The listing builds one solid part. Answer for the finished solid, in the listing's coordinates (mm). A direction names the side the tool comes from. Give positions to 0.01 mm unless a question says otherwise; leave off trailing zeros. Order: outer loops, then holes, each group sorted by start corner. A loop starts at its lowest first (then second) coordinate and runs counter-clockwise, first axis right, second up. Notation, with made-up numbers: (-9.5, -7.75) - (43.5, -7.75) arc R15 ccw to (43.5, 8.25) - close; hole circle Ø7 at (-4.5, 32.5). An arc over 180 degrees is marked (long way). Write each question's results on one line, items separated by ' | '. Start each with the question number.
1. Section C-C (x = -3) is taken. Give the vertices of the cut face in (y, z).
2. Find the intervals of material crossed by L1, parallel to X at y = 3.25, z = 9.5; L2, parallel to Z at x = 15, y = 13.5; L3, parallel to Y at x = 59, z = 8, in increasing order.
3. Which of the six approach directions +Z, -Z, +X, -X, +Y, -Y give full straight-line access (tool end or side, diameter ignored) to faces 4 (the face through (18, -7.857, 7)), 5 (the face through (38, 12.143, 7)), 6 (the face through (53.44, 2, 7))?
4. Section A-A (z = 8.5) is taken. Give the vertices of the cut face in (x, y), and give its area (3 significant figures).
5. Flat-ended cylindrical pins translate along their axes: pin 1 (5.5 mm diameter, centred on y = 0, z = 7.5, fed in from +X); pin 2 (1 mm diameter, centred on y = -8, z = 6.5, fed in from -X); pin 3 (4 mm diameter, centred on x = -10.5, y = 7, fed in from +Z); pin 4 (5.5 mm diameter, centred on x = -21, z = 8, fed in from -Y). Find the tip coordinate at first contact, or state that the pin passes through.
6. Section D-D (x = 52) is taken. Give the vertices of the cut face in (y, z).
7. Determine the mould class of faces 1 (the face through (7, 4, 5)), 2 (the face through (-2, 12.143, 7)), 3 (the face through (68.44, 4, 2)) for opening direction X: released by +X, released by -X, zero draft, split by the parting line, or undercut.
8. Section B-B (y = 3) is taken. Give the vertices of the cut face in (x, z), and give its area (3 significant figures).
from build123d import *

# Parameters (mm, degrees)
SKETCH1_W           = 100
SKETCH1_H           = 30
BOSS_EXTRUDE1_DEPTH = 5
SKETCH2_W           = 10
SKETCH2_H           = 20
BOSS_EXTRUDE2_DEPTH = 5
LPATTERN1_COUNT     = 5
LPATTERN1_PITCH     = 20


with BuildPart() as part:
    # Sketch1 → Boss-Extrude1 (new body)
    with BuildSketch(Plane.XY):
        with Locations((18.440366972, 3.71559633)):
            Rectangle(SKETCH1_W, SKETCH1_H)
    extrude(amount=BOSS_EXTRUDE1_DEPTH)

    # Sketch2 → Boss-Extrude2 (add)
    with BuildSketch(Plane.XY.offset(5)):
        with Locations((-21.559633028, 2.143304858)):
            Rectangle(SKETCH2_W, SKETCH2_H)
    boss_extrude2 = extrude(amount=BOSS_EXTRUDE2_DEPTH)

    # LPattern1: Boss-Extrude2 ×5
    with Locations(*[(i * LPATTERN1_PITCH, 0, 0) for i in range(1, LPATTERN1_COUNT)]):
        add(boss_extrude2)


solid = part.part
Reported:
1) outline: (-11.28, 0) - (18.72, 0) - (18.72, 5) - (12.14, 5) - (12.14, 10) - (-7.86, 10) - (-7.86, 5) - (-11.28, 5) - close
2) L1: -26.56 to -16.56, -6.56 to 3.44, 13.44 to 23.44, 33.44 to 43.44, 53.44 to 63.44 | L2: 0 to 5 | L3: -7.86 to 12.14
3) face 4: +Z, +X, -X, -Y | face 5: +Z, +X, -X, +Y | face 6: +Z, +Y, -Y
4) outline: (-26.56, -7.86) - (-16.56, -7.86) - (-16.56, 12.14) - (-26.56, 12.14) - close; (-6.56, -7.86) - (3.44, -7.86) - (3.44, 12.14) - (-6.56, 12.14) - close; (13.44, -7.86) - (23.44, -7.86) - (23.44, 12.14) - (13.44, 12.14) - close; (33.44, -7.86) - (43.44, -7.86) - (43.44, 12.14) - (33.44, 12.14) - close; (53.44, -7.86) - (63.44, -7.86) - (63.44, 12.14) - (53.44, 12.14) - close | area: 1,000 mm²
5) pin 1: x = 68.44 | pin 2: x = -26.56 | pin 3: z = 5 | pin 4: y = -7.86
6) outline: (-11.28, 0) - (18.72, 0) - (18.72, 5) - (-11.28, 5) - close
7) face 1: undercut | face 2: zero draft | face 3: released by +X
8) outline: (-31.56, 0) - (68.44, 0) - (68.44, 5) - (63.44, 5) - (63.44, 10) - (53.44, 10) - (53.44, 5) - (43.44, 5) - (43.44, 10) - (33.44, 10) - (33.44, 5) - (23.44, 5) - (23.44, 10) - (13.44, 10) - (13.44, 5) - (3.44, 5) - (3.44, 10) - (-6.56, 10) - (-6.56, 5) - (-16.56, 5) - (-16.56, 10) - (-26.56, 10) - (-26.56, 5) - (-31.56, 5) - close | area: 750 mm²
